Work out the finished part from the listing and answer in its coordinate system (mm). A direction names the side the tool comes from. Coordinates: 2 decimals unless noted, no trailing zeros. Loops run counter-clockwise (first coordinate to the right, second up) from the corner with the lowest first, then second, coordinate; pieces in that order, holes last. Notation, with made-up numbers: M -34,-38 L -23,-38 A21 cw -23,-32 Z; hole C -11.75,41.5 d8. An arc over 180 degrees is marked long. Write each question's results on one line, items separated by ' | '.
Solid Edge part; units mm, degrees
sketch "Sketch1" plane through (0, 0, 0) normal (0, -1, 0) x (1, 0, 0)
  line L0 (325, 325) -> (0, 325)
  line L1 (0, 0) -> (0, 325)
  line L2 (0, 0) -> (325, 0)
  line L3 (325, 0) -> (325, 325)
extrude "Protrusion1" add sketch "Sketch1" against normal blind 100
sketch "Sketch2" plane through (0, 50, 162.5) normal (-1, 0, 0) x (0, -1, 0)
  line L0 (-50, 162.5) -> (-50, -62.5)
  line L1 (-50, -62.5) -> (50, -62.5)
  line L2 (50, -62.5) -> (50, 162.5)
  line L3 (50, 162.5) -> (-50, 162.5)
  dimension "D1" = 50
extrude "Extrusionsausschnitt_1" cut sketch "Sketch2" against normal blind 100
sketch "Sketch3" plane through (0, 50, 50) normal (-1, 0, 0) x (0, -1, 0)
  line L0 (30, 30) -> (50, 30)
  line L1 (50, 50) -> (50, 30)
  line L2 (-50, 50) -> (50, 50)
  line L3 (-50, 30) -> (-50, 50)
  line L4 (-50, 30) -> (-30, 30)
  line L5 (-30, 30) -> (-30, -30)
  line L6 (-30, -30) -> (-50, -30)
  line L7 (-50, -30) -> (-50, -50)
  line L8 (-50, -50) -> (50, -50)
  line L9 (50, -50) -> (50, -30)
  line L10 (50, -30) -> (30, -30)
  line L11 (30, -30) -> (30, 30)
extrude "Extrusionsausschnitt_2" cut sketch "Sketch3" against normal blind 60
sketch "Sketch4" plane through (162.5, 0, 162.5) normal (0, -1, 0) x (1, 0, 0)
  line L0 (0, -162.5) -> (162.5, 82.5)
  line L1 (162.5, 82.5) -> (162.5, -162.5)
  line L2 (162.5, -162.5) -> (0, -162.5)
  dimension "D1" = 162.5
extrude "Extrusionsausschnitt_3" cut sketch "Sketch4" against normal blind 100
sketch "Sketch5" plane through (162.5, 0, 162.5) normal (0, -1, 0) x (1, 0, 0)
  line L0 (86.7347, 162.5) -> (-62.5, -62.5)
  line L1 (-62.5, 162.5) -> (-62.5, -62.5)
  line L2 (86.7347, 162.5) -> (-62.5, 162.5)
extrude "Extrusionsausschnitt_4" cut sketch "Sketch5" against normal blind 100
hole "Bohrung_1" at (260, 0, 245) direction (0, 1, 0) diameter 20 end up to next
sketch "Sketch6" plane through (162.5, 0, 162.5) normal (0, -1, 0) x (1, 0, 0)
  arc A0 (162.5, 82.5) -> (64.2476, 138.3505) centre (97.5, 82.5) ccw
  line L0 (64.2476, 138.3505) -> (74.5932, 173.0121)
  line L1 (74.5932, 173.0121) -> (182.984, 173.0121)
  line L2 (182.984, 173.0121) -> (182.984, 82.5)
  line L3 (182.984, 82.5) -> (162.5, 82.5)
extrude "Extrusionsausschnitt_5" cut sketch "Sketch6" against normal blind 1030.7855
hole "Bohrung_2" at (10, 0, 70) direction (0, 1, 0) diameter 10.5 end up to next start chamfer 1 start chamfer angle 45
hole "Hole1" at (50, 0, 30) direction (0, 1, 0) diameter 10.5 end up to next start chamfer 1 start chamfer angle 45
hole "Bohrung_4" at (50, 100, 70) direction (0, -1, 0) diameter 10.5 end up to next start chamfer 1 start chamfer angle 45
hole "Hole2" at (10, 100, 30) direction (0, -1, 0) diameter 10.5 end up to next start chamfer 1 start chamfer angle 45
1) For a pull along Z with two mould halves and no side action, classify faces 1 (the face through (60, 49, 51)), 2 (the face through (53.55, 10.37, 33.87)), 3 (the face through (242.612, 49.3, 120.785)) as released by +Z, released by -Z, zero draft, split by the parting line, or undercut.
Check result:
face 1: zero draft | face 2: undercut | face 3: released by -Z
2) Find section D-D, the plane z = 70. Give the vertices of the cut face in (x, y), and give its area (3 significant figures).
Check result:
outline: M 0,0 L 3.75,0 L 4.75,1 L 4.75,20 L 0,20 Z; M 0,80 L 44.75,80 L 44.75,99 L 43.75,100 L 0,100 Z; M 15.25,1 L 16.25,0 L 208.93,0 L 208.93,100 L 56.25,100 L 55.25,99 L 55.25,80 L 60,80 L 60,20 L 15.25,20 Z | area: 16,900 mm^2
3) Straight lines are drawn through the part: probe 1 along Z at (x, y) = (50, 12); probe 2 along Y at (x, z) = (56, 48); probe 3 along Z at (x, y) = (92, 36.5). For each, find the intervals that lie inside material, in ascending order. Write a range as [from, to].
Check result:
probe 1: [20, 24.75], [35.25, 80] | probe 2: [0, 20], [80, 100] | probe 3: [0, 100]
4) Which of the six approach directions +Z, -Z, +X, -X, +Y, -Y give full straight-line access (tool end or side, diameter ignored) to faces 4 (the face through (30, 10, 80)), 5 (the face through (13.55, 10.37, 73.87)), 6 (the face through (30, 10, 20)), 7 (the face through (111, 49, 0))?
Check result:
face 4: +Z, -X, +Y, -Y | face 5: -Y | face 6: -Z, -X, +Y, -Y | face 7: -Z, +X, -X, +Y, -Y
5) Find section B-B, the plane x = 260. Give the vertices of the cut face in (y, z), and give its area (3 significant figures).
Check result:
outline: M 0,147 L 100,147 L 100,235 L 0,235 Z; M 0,255 L 100,255 L 100,310 L 0,310 Z | area: 14,300 mm^2
6) Find section A-A, the plane x = 50. Give the vertices of the cut face in (y, z), and give its area (3 significant figures).
Check result:
outline: M 0,20 L 20,20 L 20,24.75 L 1,24.75 L 0,23.75 Z; M 0,36.25 L 1,35.25 L 20,35.25 L 20,80 L 0,80 Z; M 80,20 L 100,20 L 100,63.75 L 99,64.75 L 80,64.75 Z; M 80,75.25 L 99,75.25 L 100,76.25 L 100,80 L 80,80 Z | area: 1,980 mm^2
7) Find section C-C, the plane y = 91. Give the vertices of the cut face in (x, z).
Check result:
outline: M 0,20 L 60,20 L 60,0 L 162.5,0 L 325,245 A65 ccw 236.32,305.53 L 100,100 L 60,100 L 60,80 L 0,80 Z; hole C 10,30 d10.5; hole C 50,70 d10.5; hole C 260,245 d20
8) Given pin 1 Ø6.5 at (x, z) = (50, 30) entering from -Y; pin 2 Ø8 at (x, y) = (278.5, 79) entering from -Z; pin 3 Ø3 at (x, y) = (268.5, 21) entering from -Z, each flat-ended and moving along its own axis, determine where each tip first touches the part or whether it passes through.
Check result:
pin 1: y = 80 | pin 2: z = 168.86 | pin 3: z = 157.55
